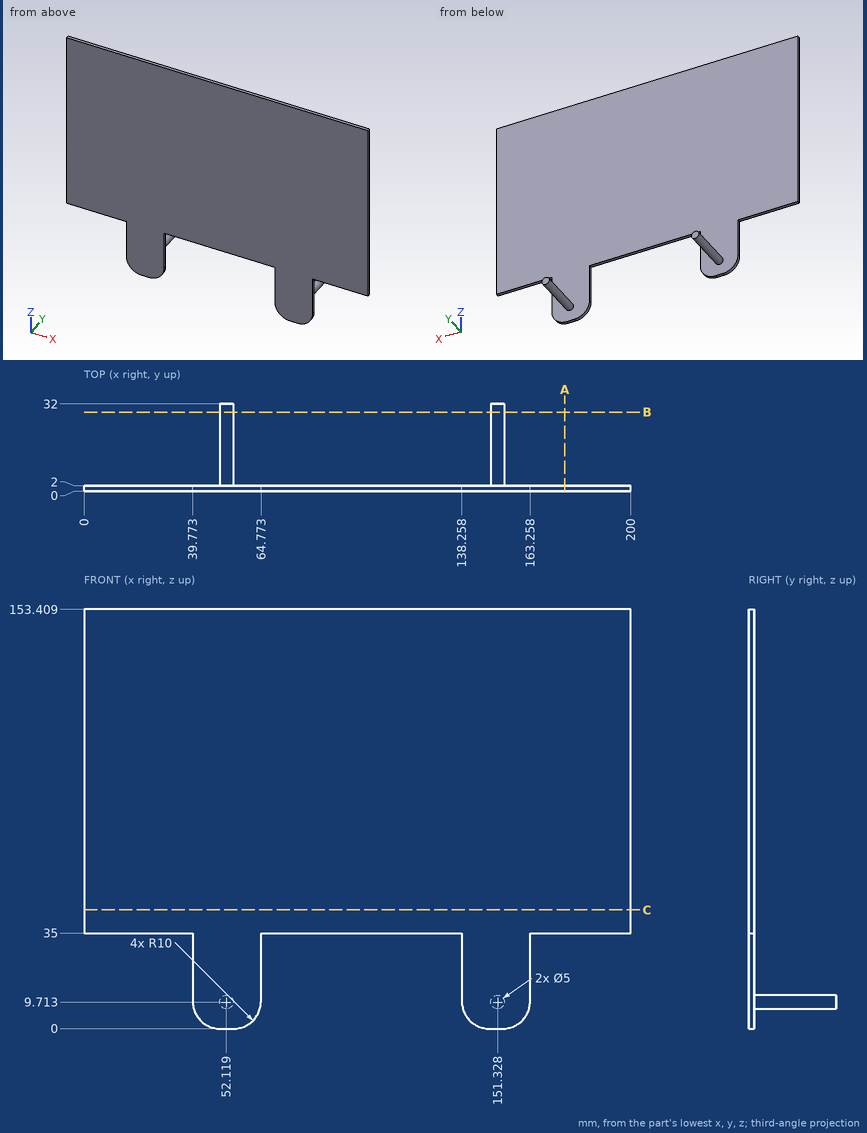
Input: dimensioned drawing with shaded views. Units: mm. Origin: part minimum x, y, z. Give positions to 0.01 mm unless a question says otherwise; leave off trailing zeros. Write each loop counter-clockwise with the first axis right and the second up, starting at its lowest first coordinate (ties: lowest second). Pieces come first, ordered by that corner, then holes.
1. Material intervals for line 1 along Y through (x, z) = (25, 98); line 2 along Z through (x, y) = (121.5, 1); line 3 along Z through (x, y) = (53.5, 6.5), sorted ascending.
2. Section query C-C (z = 43.5). Return the cut outline in (x, y), then the cut area to 3 significant figures.
3. First-contact query: pin 1 (8 mm diameter, centred on x = 171.5, z = 82.5, fed in from +Y); pin 2 (1.6 mm diameter, centred on x = 18.5, y = 1.5, fed in from -Z); pin 3 (2 mm diameter, centred on y = 1, z = 26, fed in from -X); pin 4 (2 mm diameter, centred on x = 109, z = 84.5, fed in from -Y). Flat tips, straight axial feed; report the tip coordinate or a pass-through.
4. Section query B-B (y = 29). Return the cut outline in (x, z).
5. Section query A-A (x = 176). Return the cut outline in (y, z).
Output values:
1. line 1: y = 0 to 2
1. line 2: z = 35 to 153.41
1. line 3: z = 7.63 to 11.8
2. outline: (0, 0) - (200, 0) - (200, 2) - (0, 2) - close
2. area: 400 mm2
3. pin 1: stops at y = 2
3. pin 2: stops at z = 35
3. pin 3: stops at x = 39.77
3. pin 4: stops at y = 0
4. outline: circle Ø5 at (52.12, 9.71); circle Ø5 at (151.33, 9.71)
5. outline: (0, 35) - (2, 35) - (2, 153.41) - (0, 153.41) - close
